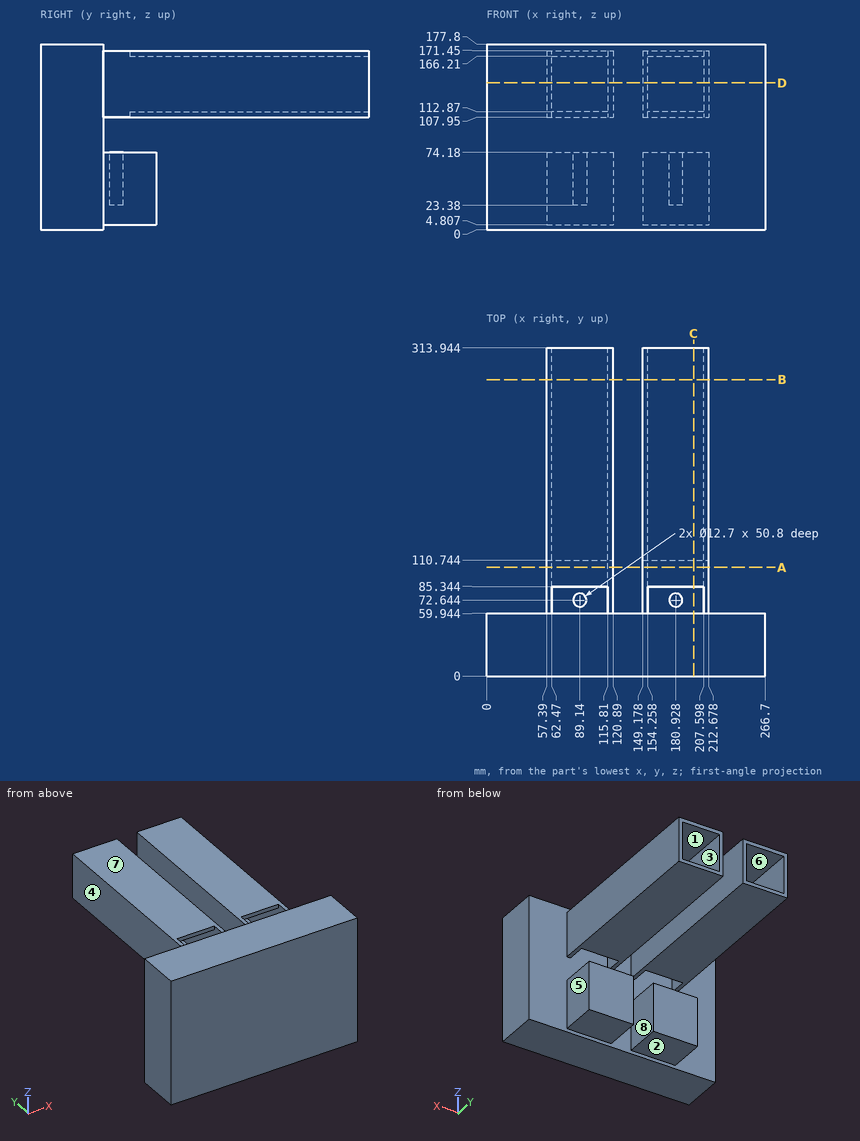
Part print with two shaded views. Sizes in mm from the minimum x, y, z corner. A direction names the side the tool comes from. Round coordinates to 2 decimals unless told otherwise and drop trailing zeros. Order: outer loops, then holes, each group sorted by start corner. A loop starts at its lowest first (then second) coordinate and runs counter-clockwise, first axis right, second up. Notation, with made-up numbers: (45, 30) -> (84, 30) arc R23 cw to (84, 54) -> close; hole circle Ø9 at (0.25, 54.25). An arc over 180 degrees is marked (long way). Use one line per item in the form item = value.
Item 1: Cut at D-D, the plane z = 140.5. Write the cut outline in (x, y), and give its area (4 significant figures).
Returned:
outline = (0, 0) -> (266.7, 0) -> (266.7, 59.94) -> (212.68, 59.94) -> (212.68, 313.94) -> (207.6, 313.94) -> (207.6, 59.94) -> (154.26, 59.94) -> (154.26, 313.94) -> (149.18, 313.94) -> (149.18, 59.94) -> (120.89, 59.94) -> (120.89, 313.94) -> (115.81, 313.94) -> (115.81, 59.94) -> (62.47, 59.94) -> (62.47, 313.94) -> (57.39, 313.94) -> (57.39, 59.94) -> (0, 59.94) -> close
area = 21,150 mm^2
Item 2: Cut at C-C, the plane x = 198. Write the cut outline in (y, z), and give its area (3 significant figures).
Returned:
outline = (0, 0) -> (59.94, 0) -> (59.94, 4.81) -> (110.74, 4.81) -> (110.74, 74.18) -> (59.94, 74.18) -> (59.94, 177.8) -> (0, 177.8) -> close; (85.34, 107.95) -> (313.94, 107.95) -> (313.94, 112.87) -> (85.34, 112.87) -> close; (85.34, 166.21) -> (313.94, 166.21) -> (313.94, 171.45) -> (85.34, 171.45) -> close
area = 16,500 mm^2
Item 3: Flat gauge pins, fed straight in: pin 1 Ø12 at (x, y) = (186.5, 83.5) entering from -Z; pin 2 Ø12 at (y, z) = (85.5, 116) entering from +X; pin 3 Ø10 at (x, z) = (129, 53.5) entering from +Y. Where does each tip first touch, or does it go through?
Returned:
pin_1 = 4.81
pin_2 = 212.68
pin_3 = 59.94
Item 4: Cut at A-A, the plane y = 104. Write the cut outline in (x, z), and give its area (3 significant figures).
Returned:
outline = (57.39, 4.81) -> (120.89, 4.81) -> (120.89, 74.18) -> (57.39, 74.18) -> close; (57.39, 107.95) -> (120.89, 107.95) -> (120.89, 171.45) -> (57.39, 171.45) -> close; (149.18, 4.81) -> (212.68, 4.81) -> (212.68, 74.18) -> (149.18, 74.18) -> close; (149.18, 107.95) -> (212.68, 107.95) -> (212.68, 171.45) -> (149.18, 171.45) -> close; hole (62.47, 112.87) -> (115.81, 112.87) -> (115.81, 166.21) -> (62.47, 166.21) -> close; hole (154.26, 112.87) -> (207.6, 112.87) -> (207.6, 166.21) -> (154.26, 166.21) -> close
area = 11,200 mm^2
Item 5: Cut at B-B, the plane y = 283.5. Write the cut outline in (x, z).
Returned:
outline = (57.39, 107.95) -> (120.89, 107.95) -> (120.89, 171.45) -> (57.39, 171.45) -> close; (149.18, 107.95) -> (212.68, 107.95) -> (212.68, 171.45) -> (149.18, 171.45) -> close; hole (62.47, 112.87) -> (115.81, 112.87) -> (115.81, 166.21) -> (62.47, 166.21) -> close; hole (154.26, 112.87) -> (207.6, 112.87) -> (207.6, 166.21) -> (154.26, 166.21) -> close
Item 6: Tool access for the marked faces 5, 6, 7 and 8: list every direction of +Z, -Z, +X, -X, +Y, -Y with a clear straight run to the whole face (end or side of a thin tool).
Returned:
face_5 = +Z, -Z, +X, +Y
face_6 = +Y
face_7 = +Z, +X, -X, +Y
face_8 = +Z, -Z, +Y
Item 7: Pull direction X, two halves, no side cores. Call the marked faces 1, 2, 3 and 4: released by +X, released by -X, zero draft, split by the parting line, or undercut.
Returned:
face_1 = undercut
face_2 = zero draft
face_3 = undercut
face_4 = released by -X
Item 8: Drill centre lines: line 1 (X direction, y = 80, z = 133.5); line 2 (Z direction, x = 166, y = 118.5); line 3 (X direction, y = 99.5, z = 30.5). Where is each one in solid material? Low to high.
Returned:
line_1 = 57.39 to 62.47, 115.81 to 120.89, 149.18 to 154.26, 207.6 to 212.68
line_2 = 107.95 to 112.87, 166.21 to 171.45
line_3 = 57.39 to 120.89, 149.18 to 212.68
